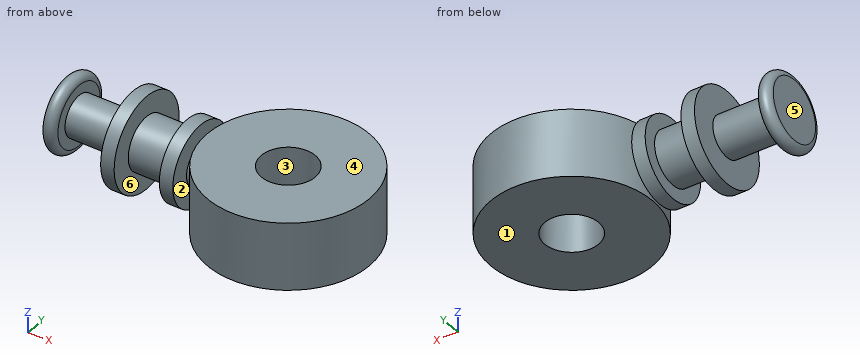
from build123d import *

# Parameters (mm, degrees)
SKETCH1_R                = 9.4107
SKETCH1_R_2              = 3.1369
BOSS_EXTRUDE1_DEPTH      = 3.92049
BOSS_EXTRUDE1_DEPTH_BACK = 3.92049


with BuildPart() as part:
    # Sketch1 → Boss-Extrude1 (new body, two sides)
    with BuildSketch(Plane.XY) as boss_extrude1_sk:
        Circle(SKETCH1_R)
        Circle(SKETCH1_R_2, mode=Mode.SUBTRACT)
    extrude(amount=BOSS_EXTRUDE1_DEPTH)
    extrude(boss_extrude1_sk.sketch, amount=-BOSS_EXTRUDE1_DEPTH_BACK)

    # Sketch2 → Revolve1 (revolve)
    with BuildSketch(Plane(origin=(0, 0, 0), x_dir=(1, 0, 0), z_dir=(0, 1, 0))):
        with BuildLine():
            Line((-5.959188984, 0), (-25.87498, 0))
            Line((-25.87498, 0), (-25.87498, 3.52933))
            ThreePointArc((-25.87498, 3.52933), (-25.09139, 4.31292), (-24.3078, 3.52933))
            Line((-24.3078, 3.52933), (-24.3078, 2.35204))
            Line((-24.3078, 2.35204), (-18.034, 2.35204))
            Line((-18.034, 2.35204), (-18.034, 5.41528))
            Line((-18.034, 5.41528), (-16.46428, 5.41528))
            Line((-16.46428, 5.41528), (-16.46428, 3.06197))
            Line((-16.46428, 3.06197), (-11.7602, 3.06197))
            Line((-11.7602, 3.06197), (-11.7602, 4.63042))
            Line((-11.7602, 4.63042), (-10.19302, 4.63042))
            Line((-10.19302, 4.63042), (-10.19302, 2.35204))
            Line((-10.19302, 2.35204), (-5.959188984, 2.35204))
            Line((-5.959188984, 2.35204), (-5.959188984, 0))
        make_face()
    revolve(axis=Axis((-5.959188984, 0, 0), (-1, 0, 0)))


solid = part.part
Verification items for the finished model (mm, model axes). Face numbers are marked on the shaded views. A direction names the side the tool comes from. Give positions to 0.01 mm unless a question says otherwise; leave off trailing zeros. Write each loop counter-clockwise with the first axis right and the second up, starting at its lowest first coordinate (ties: lowest second). Pieces come first, ordered by that corner, then holes. Notation, with made-up numbers: M 38,32.25 L 85,32.25 A24 ccw 85,53.25 Z; hole C 51.5,4 d8. An arc over 180 degrees is marked long. Put each result on its own line as item: value. Start each with the question number.
1. Set-up check for the marked faces 1, 2 and 3: record each of +Z, -Z, +X, -X, +Y, -Y from which the full face is reachable in a straight line by a thin tool's end or side.
2. Section check D-D (x = -22). Record the cut outline in (y, z), and give its area (3 significant figures).
3. Draft check along X on the marked faces 4, 5 and 6. Enter one of: +X half, -X half, draft (parallel to the pull), parting line (faces both ways), or undercut.
4. Section check C-C (z = 0). Record the cut outline in (x, y), and give its area (3 significant figures).
5. Scan lines: line 1 along Y through (x, z) = (0, -1.75); line 2 along Z through (x, y) = (-18.5, 0); line 3 along Z through (x, y) = (4.5, -7.5). Record each from-to range of solid material in increasing order. Write a range as [from, to].
6. Go/stop test with flat-tipped pins: pin 1 Ø4 at (x, y) = (-8.5, -2.5) entering from +Z; pin 2 Ø6 at (x, y) = (-10.5, 6.5) entering from -Z; pin 3 Ø3 at (y, z) = (7, 0) entering from +X. Record where each tip stops, or that it passes through.
7. Section check A-A (x = 0). Record the cut outline in (y, z), and give its area (3 significant figures).
Answer list:
1. face 1: -Z, +X, +Y, -Y
1. face 2: none
1. face 3: +Z, -Z
2. outline: C 0,0 d4.7
2. area: 17.4 mm2
3. face 4: draft
3. face 5: -X half
3. face 6: undercut
4. outline: M -25.87,-3.53 A0.78 ccw -24.31,-3.53 L -24.31,-2.35 L -18.03,-2.35 L -18.03,-5.42 L -16.46,-5.42 L -16.46,-3.06 L -11.76,-3.06 L -11.76,-4.63 L -10.19,-4.63 L -10.19,-2.35 L -9.11,-2.35 A9.41 ccw long -9.11,2.35 L -10.19,2.35 L -10.19,4.63 L -11.76,4.63 L -11.76,3.06 L -16.46,3.06 L -16.46,5.42 L -18.03,5.42 L -18.03,2.35 L -24.31,2.35 L -24.31,3.53 A0.78 ccw -25.87,3.53 Z; hole C 0,0 d6.27
4. area: 354 mm2
5. line 1: [-9.41, -3.14], [3.14, 9.41]
5. line 2: [-2.35, 2.35]
5. line 3: [-3.92, 3.92]
6. pin 1: z = 4.4
6. pin 2: z = -3.92
6. pin 3: x = 7.64
7. outline: M -9.41,-3.92 L -3.14,-3.92 L -3.14,3.92 L -9.41,3.92 Z; M 3.14,-3.92 L 9.41,-3.92 L 9.41,3.92 L 3.14,3.92 Z
7. area: 98.4 mm2
